from build123d import *

# Parameters (mm, degrees)
BOSS_EXTRUDE1_DEPTH = 15
SKETCH2_R           = 7.5
BOSS_EXTRUDE2_DEPTH = 10
SKETCH3_R           = 6
CUT_EXTRUDE1_DEPTH  = 2
BOSS_EXTRUDE3_DEPTH = 3


with BuildPart() as part:
    # Sketch1 → Boss-Extrude1 (new body)
    with BuildSketch(Plane.XY):
        with BuildLine():
            Line((1, 0), (44, 0))
            ThreePointArc((44, 0), (44.707106781, 0.292893219), (45, 1))
            Line((45, 1), (45, 19))
            ThreePointArc((45, 19), (44.707106781, 19.707106781), (44, 20))
            Line((44, 20), (1, 20))
            ThreePointArc((1, 20), (0.292893219, 19.707106781), (0, 19))
            Line((0, 19), (0, 1))
            ThreePointArc((0, 1), (0.292893219, 0.292893219), (1, 0))
        make_face()
    extrude(amount=BOSS_EXTRUDE1_DEPTH)

    # Sketch2 → Boss-Extrude2 (add)
    with BuildSketch(Plane.XY.offset(15)):
        with Locations(Location((10, 10, 0), (0, 0, 180))):
            Circle(SKETCH2_R)
        with Locations(Location((35, 10, 0), (0, 0, 180))):
            Circle(SKETCH2_R)
    extrude(amount=BOSS_EXTRUDE2_DEPTH)

    # Sketch3 → Cut-Extrude1 (cut)
    with BuildSketch(Plane.XY.offset(25)):
        with Locations((10, 10)):
            Circle(SKETCH3_R)
        with Locations((35, 10)):
            Circle(SKETCH3_R)
    extrude(amount=-CUT_EXTRUDE1_DEPTH, mode=Mode.SUBTRACT)

    # Sketch4 → Boss-Extrude3 (add)
    with BuildSketch(Plane.XY.offset(15)):
        with BuildLine():
            Line((18.5, 4), (26.5, 4))
            ThreePointArc((26.5, 4), (27.207106781, 3.707106781), (27.5, 3))
            Line((27.5, 3), (27.5, 2))
            ThreePointArc((27.5, 2), (27.207106781, 1.292893219), (26.5, 1))
            Line((26.5, 1), (18.5, 1))
            ThreePointArc((18.5, 1), (17.792893219, 1.292893219), (17.5, 2))
            Line((17.5, 2), (17.5, 3))
            ThreePointArc((17.5, 3), (17.792893219, 3.707106781), (18.5, 4))
        make_face()
    extrude(amount=BOSS_EXTRUDE3_DEPTH)


solid = part.part
The model under review builds one solid part; all positions refer to its coordinate system, in mm. A direction names the side the tool comes from. Coordinates: 2 decimals unless noted, no trailing zeros. Loops run counter-clockwise (first coordinate to the right, second up) from the corner with the lowest first, then second, coordinate; pieces in that order, holes last.
(1) Tool access review of faces 5 (the flat face through (23, 3, 18)), 6 (the flat face through (17.5, 2.5, 16.5)), 7 (the cylindrical face through (27.215, 1.301, 16.479)), 8 (the flat face through (22, 10, 15)): name each direction out of +Z, -Z, +X, -X, +Y, -Y from which nothing blocks a thin tool from reaching the whole face with its end or side.
Determined:
face 5: +Z, +Y, -Y
face 6: +Z, -Y
face 7: +Z, +X, -Y
face 8: +Z
(2) Insertion check: P1, Ø3.5, axis at x = 12, y = 8.5, coming from the +Z side; P2, Ø1.1, axis at y = 2.5, z = 16, coming from the +X side; P3, Ø0.9, axis at x = 21.5, y = 2.5, coming from the +Z side. Each pin has a flat end and moves straight along its axis. Give the tip position at first contact, or say it passes through.
Determined:
P1: stops at z = 23
P2: stops at x = 37.82
P3: stops at z = 18
(3) Consider section D-D, the plane y = 5.5. Give the boundary of the cut face in (x, z), plus the area to 3 significant figures.
Determined:
outline: (0, 0) - (45, 0) - (45, 15) - (41, 15) - (41, 25) - (38.97, 25) - (38.97, 23) - (31.03, 23) - (31.03, 25) - (29, 25) - (29, 15) - (16, 15) - (16, 25) - (13.97, 25) - (13.97, 23) - (6.03, 23) - (6.03, 25) - (4, 25) - (4, 15) - (0, 15) - close
area: 883 mm2
(4) Consider section A-A, the plane z = 16.5. Give the boundary of the cut face in (x, y), plus the area to 3 significant figures.
Determined:
outline: circle Ø15 at (10, 10); (17.5, 2) arc R1 ccw to (18.5, 1) - (26.5, 1) arc R1 ccw to (27.5, 2) - (27.5, 3) arc R1 ccw to (26.5, 4) - (18.5, 4) arc R1 ccw to (17.5, 3) - close; circle Ø15 at (35, 10)
area: 383 mm2
(5) Consider section C-C, the plane x = 10. Give the boundary of the cut face in (y, z).
Determined:
outline: (0, 0) - (20, 0) - (20, 15) - (17.5, 15) - (17.5, 25) - (16, 25) - (16, 23) - (4, 23) - (4, 25) - (2.5, 25) - (2.5, 15) - (0, 15) - close
(6) Wall thickness on L1, parallel to Y at x = 35, z = 23.9; L2, parallel to Z at x = 19, y = 2.25; L3, parallel to Z at x = 26, y = 12.5: over which ranges is each line inside the solid? List them lowest first.
Determined:
L1: y = 2.5 to 4, 16 to 17.5
L2: z = 0 to 18
L3: z = 0 to 15
(7) Consider section B-B, the plane y = 10. Give the boundary of the cut face in (x, z).
Determined:
outline: (0, 0) - (45, 0) - (45, 15) - (42.5, 15) - (42.5, 25) - (41, 25) - (41, 23) - (29, 23) - (29, 25) - (27.5, 25) - (27.5, 15) - (17.5, 15) - (17.5, 25) - (16, 25) - (16, 23) - (4, 23) - (4, 25) - (2.5, 25) - (2.5, 15) - (0, 15) - close
(8) Draft analysis for pull direction Y (two halves, no side actions). For faces 1 (the flat face through (33, 4, 25)), 2 (the flat face through (23, 20, 7)), 3 (the flat face through (10, 10, 23)), 4 (the cylindrical face through (8.699, 4.143, 24.014)), state which applies: +Y half, -Y half, draft (parallel to the pull), parting line (faces both ways), or undercut.
Determined:
face 1: draft
face 2: +Y half
face 3: undercut
face 4: undercut
